from build123d import *

# Parameters (mm, degrees)
F1_DEPTH = 20
F2_W     = 8.5
F2_H     = 20
F3_DEPTH = 3


with BuildPart() as f1:
    # F0 (on Top) → F1 (new body)
    with BuildSketch(Plane.XY):
        with BuildLine():
            ThreePointArc((-51.423708, -10), (-52.387, 0), (-51.423708, 10))
            Line((-51.423708, 10), (-55.387, 10))
            Line((-55.387, 10), (-55.387, 0))
            Line((-55.387, 0), (-55.387, -10))
            Line((-55.387, -10), (-51.423708, -10))
        make_face()
    extrude(amount=F1_DEPTH)

    # F2 (on face) → F3 (join)
    with BuildSketch(Plane(origin=(-55.387, 0, 0), x_dir=(0, -1, 0), z_dir=(-1, 0, 0))):
        with Locations((5.75, 10)):
            Rectangle(F2_W, F2_H)
        with Locations((-5.75, 10)):
            Rectangle(F2_W, F2_H)
    extrude(amount=F3_DEPTH)


solid = f1.part
Work out the finished part from the listing and answer in its coordinate system (mm). A direction names the side the tool comes from. Coordinates: 2 decimals unless noted, no trailing zeros. Write each loop counter-clockwise with the first axis right and the second up, starting at its lowest first coordinate (ties: lowest second). Pieces come first, ordered by that corner, then holes. Notation, with made-up numbers: M 89.5,-11 L 140.5,-11 A20 ccw 140.5,22 Z; hole C 7,-11.75 d6. An arc over 180 degrees is marked long. Write item = value, one per line.
1. Determine the mould class of faces 1 (the face through (-58.387, -6, 10)), 2 (the face through (-55, -10, 10)), 3 (the face through (-52.387, -0.141, 9.86)), 4 (the face through (-57, 1.5, 10)) for opening direction Y: released by +Y, released by -Y, zero draft, split by the parting line, or undercut.
Solution:
face_1 = zero draft
face_2 = released by -Y
face_3 = undercut
face_4 = undercut
2. For faces 5 (the face through (-58.387, 6, 10)), 6 (the face through (-55.387, 0, 10)), determine the directions among +Z, -Z, +X, -X, +Y, -Y from which every point of the face is accessible in a straight line to the end or side of a thin tool.
Solution:
face_5 = +Z, -Z, -X, +Y, -Y
face_6 = +Z, -Z, -X
3. Flat-ended cylindrical pins translate along their axes: pin 1 (0.9 mm diameter, centred on y = 0, z = 9, fed in from -X); pin 2 (4 mm diameter, centred on y = -7, z = 14, fed in from +X); pin 3 (10 mm diameter, centred on y = 0.5, z = 4, fed in from +X). Find the tip coordinate at first contact, or state that the pin passes through.
Solution:
pin_1 = -55.39
pin_2 = -51.61
pin_3 = -52.1
4. The part is cut by section B-B (z = 2). Determine the outline of the cut face in (x, y).
Solution:
outline = M -58.39,-10 L -51.42,-10 A52.39 cw -51.42,10 L -58.39,10 L -58.39,1.5 L -55.39,1.5 L -55.39,-1.5 L -58.39,-1.5 Z
5. The part is cut by section C-C (y = -1). Determine the outline of the cut face in (x, z).
Solution:
outline = M -55.39,0 L -52.38,0 L -52.38,20 L -55.39,20 Z
6. The part is cut by section D-D (y = 8). Determine the outline of the cut face in (x, z).
Solution:
outline = M -58.39,0 L -51.77,0 L -51.77,20 L -58.39,20 Z
7. Straight lines are drawn through the part: line 1 (Y direction, x = -56.75, z = 1.25); line 2 (X direction, y = 2, z = 15.5); line 3 (X direction, y = 6.5, z = 4.75). For each, find the intervals that lie inside material, in ascending order. Write a range as from..to.
Solution:
line_1 = -10..-1.5, 1.5..10
line_2 = -58.39..-52.35
line_3 = -58.39..-51.98
8. The part is cut by section A-A (x = -57.5). Determine the outline of the cut face in (y, z).
Solution:
outline = M -10,0 L -1.5,0 L -1.5,20 L -10,20 Z; M 1.5,0 L 10,0 L 10,20 L 1.5,20 Z
